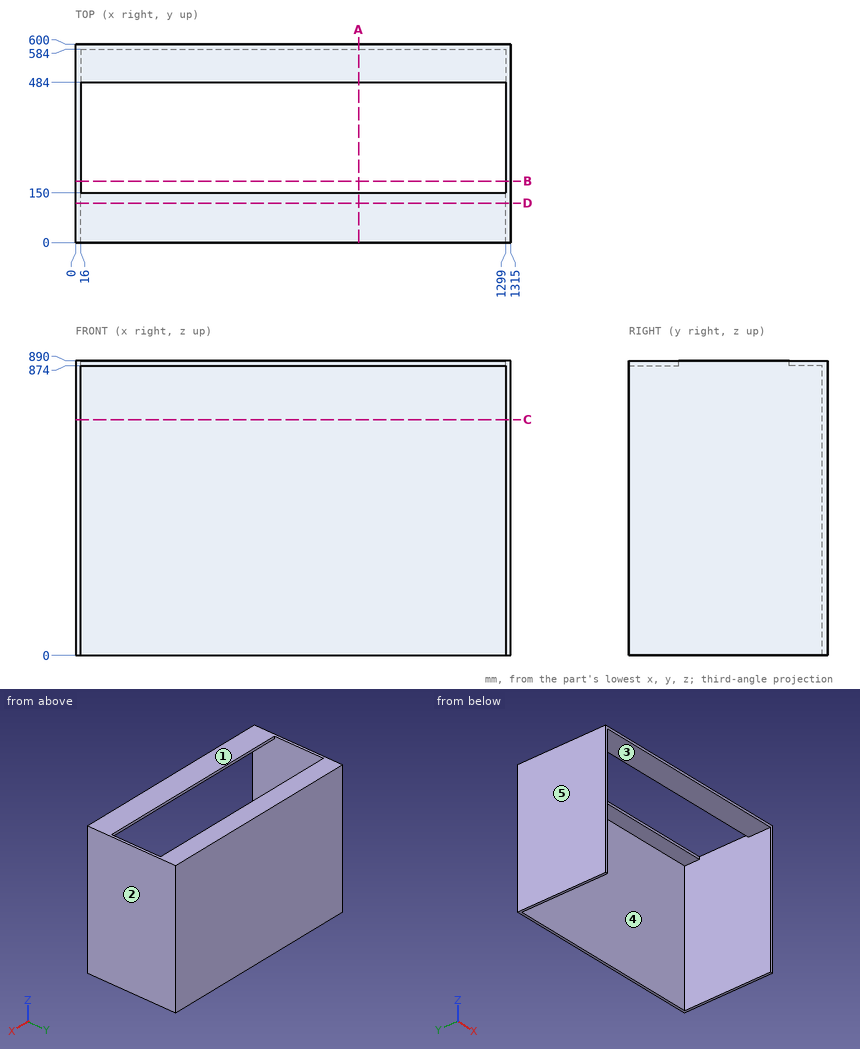
Can you work these out from the drawing? Everything is in mm from the part's minimum corner. A direction names the side the tool comes from. Give positions to 0.01 mm unless a question says otherwise; leave off trailing zeros. Write each loop counter-clockwise with the first axis right and the second up, starting at its lowest first coordinate (ties: lowest second). Pieces come first, ordered by that corner, then holes. Notation, with made-up numbers: M 29.25,66.25 L 85.25,66.25 A16 ccw 85.25,77.25 Z; hole C -1.5,28.25 d3. An arc over 180 degrees is marked long. Answer in a Markdown table with one row per item. Add a question column.
Item 1: For pin 1 Ø1.5 at (x, y) = (803, 124.5) entering from -Z; pin 2 Ø8 at (x, z) = (575.5, 885.5) entering from -Y; pin 3 Ø5 at (x, z) = (673.5, 505.5) entering from -Y, each with a flat end and sliding along its axis, tell me the tip position at first contact or that it passes through.
Item 2: On a 3-axis mill with a long thin cutter (end or side, diameter ignored), from which of +Z, -Z, +X, -X, +Y, -Y can I reach the whole of each face in a straight line? I mean the marked faces 4 and 5. Say none if no direction works.
Item 3: Imagine slicing it at D-D, the plane y = 119.5. Write out the boundary of the cut face in (x, z).
Item 4: Imagine slicing it at A-A, the plane x = 855. Write out the boundary of the cut face in (y, z).
Item 5: Imagine slicing it at B-B, the plane y = 186. Write out the boundary of the cut face in (x, z).
Item 6: Please list where these lines run through material, in increasing order: L1, parallel to X at y = 311.5, z = 301.5; L2, parallel to Y at x = 1107, z = 610; L3, parallel to Z at x = 1136, y = 498.
Item 7: Imagine slicing it at C-C, the plane z = 712. Write out the boundary of the cut face in (x, y), plus the area to 3 significant figures.
Item 8: We'd pull the mould along X, two halves only. Please class the marked faces 1, 2 and 3: released by +X, released by -X, zero draft, split by the parting line, or undercut.
Evaluation:
| question | item | result |
|---|---|---|
| 1 | pin 1 | stops at z = 874 |
| 1 | pin 2 | stops at y = 0 |
| 1 | pin 3 | stops at y = 584 |
| 2 | face 4 | -Z, -Y |
| 2 | face 5 | +Z, -Z, -X, +Y, -Y |
| 3 | outline | M 0,0 L 16,0 L 16,874 L 1299,874 L 1299,0 L 1315,0 L 1315,890 L 0,890 Z |
| 4 | outline | M 0,874 L 150,874 L 150,890 L 0,890 Z; M 484,874 L 584,874 L 584,0 L 600,0 L 600,890 L 484,890 Z |
| 5 | outline | M 0,0 L 16,0 L 16,890 L 0,890 Z; M 1299,0 L 1315,0 L 1315,890 L 1299,890 Z |
| 6 | L1 | x = 0 to 16, 1299 to 1315 |
| 6 | L2 | y = 584 to 600 |
| 6 | L3 | z = 874 to 890 |
| 7 | outline | M 0,0 L 16,0 L 16,584 L 1299,584 L 1299,0 L 1315,0 L 1315,600 L 0,600 Z |
| 7 | area | 39,700 mm² |
| 8 | face 1 | zero draft |
| 8 | face 2 | released by +X |
| 8 | face 3 | undercut |
